Autodesk Inventor part; units mm, degrees
ref_plane "Work Plane1" through (0, 11.1125, 0) normal (0, 1, 0) x (-1, 0, 0)
ref_plane "YZ Plane" through (0, 0, 0) normal (1, 0, 0) x (0, 1, 0)
ref_plane "XY Plane" through (0, 0, 0) normal (0, 0, 1) x (1, 0, 0)
sketch "Sketch1" plane through (0, 0, 0) normal (0, 0, 1) x (1, 0, 0)
  circle A0 centre (0, 0) radius 11.1125
  circle A1 centre (0, 0) radius 5.5245
  circle A2 centre (0, 0) radius 1.8415
  dimension "d0" = 22.225
  dimension "d1" = 11.049
  dimension "d2" = 3.683
extrude "Extrusion1" add sketch "Sketch1" along normal blind 10.16 contours A0
extrude "Extrusion2" add sketch "Sketch1" along normal blind 5.08 contours A1
sketch "Sketch2" plane through (0, 0, 0) normal (1, 0, 0) x (0, 1, 0)
  line L0 (11.1125, 10.16) -> (-11.1125, 10.16)
  line L1 (2.8575, 10.16) -> (-2.8575, 10.16)
  line L2 (-2.8575, 10.16) -> (-2.8575, 6.096)
  line L3 (-2.8575, 6.096) -> (2.8575, 6.096)
  line L4 (2.8575, 6.096) -> (2.8575, 10.16)
  point P0 (0, 0)
  dimension "d7" = 5.715
  dimension "d8" = 2.8575
  dimension "d9" = 4.064
extrude "Extrusion3" cut sketch "Sketch2" along normal through all
ref_plane "Work Plane1" through (0, 11.1125, 0) normal (0, 1, 0) x (-1, 0, 0)
sketch "Sketch3" plane through (0, 11.1125, 0) normal (0, 1, 0) x (-1, 0, 0)
  line L0 (11.1125, 0) -> (11.1125, 10.16) construction
  circle A0 centre (0, 2.54) radius 1.7145
  point P0 (0, 0)
  dimension "d12" = 3.429
  dimension "d13" = 2.54
extrude "Extrusion4" cut sketch "Sketch3" against normal blind 2.032
pattern_circular "Circular Pattern1" count 4 over 360 about axis through (0, 0, 0) along (0, 0, 1) of "Extrusion4"
equation "\"d5\" = 0.5 * d3"
equation "\"d10\" = 0.5 * d3"
properties part number "EncoderDisc" material "ABS Plastic"
The model under review builds one solid part; all positions refer to its coordinate system, in mm. A direction names the side the tool comes from. Coordinates: 2 decimals unless noted, no trailing zeros. Loops run counter-clockwise (first coordinate to the right, second up) from the corner with the lowest first, then second, coordinate; pieces in that order, holes last. Notation, with made-up numbers: (6.25, 81.5) -> (11.25, 81.5) arc R28 ccw to (11.25, 106.5) -> close; hole circle Ø11 at (-8.75, 71.5). An arc over 180 degrees is marked (long way). Use a Markdown table: item, result. Add a question column.
1. To check wall thickness, follow line 1 (Z direction, x = 0, y = -10.25); line 2 (Z direction, x = 10.2, y = 0); line 3 (Z direction, x = 2.25, y = 4.25). State the ranges of each line that lie inside material, in increasing order.
2. Add section C-C on y = -5.25. Write out the cut boundary in (x, z), plus the area to 3 significant figures.
3. Add section A-A on x = 0. Write out the cut boundary in (y, z), plus the area to 3 significant figures.
4. Machinability: for faces 1 (the face through (8, -2.858, 8)), 2 (the face through (-10.111, 1.713, 2.615)), 3 (the face through (-1.713, -10.111, 2.615)), 4 (the face through (10.111, -1.713, 2.615)), which of the approach directions +Z, -Z, +X, -X, +Y, -Y give a long, thin tool a straight path to every point of the face, cutting with its end or side? Answer none if there is none.
5. Clearance check with flat-ended pins moving along their axes: pin 1 Ø12 at (x, y) = (-1, -2.5) entering from +Z; pin 2 Ø6 at (x, y) = (0, 0) entering from +Z; pin 3 Ø3.5 at (x, z) = (8, 8.5) entering from -Y; pin 4 Ø1 at (y, z) = (0.5, 3) entering from +X. State where each tip first meets the part, or that it passes through.
6. Add section D-D on z = 9.5. Write out the cut boundary in (x, y) (1 decimal).
7. Add section B-B on z = 1.5. Write out the cut boundary in (x, y) (1 decimal).
8. Draft analysis for pull direction X (two halves, no side actions). For faces 5 (the face through (10.265, 4.256, 5.009)), 6 (the face through (0, 9.08, 3)), 7 (the face through (-5.2, -2.3, 10.16)), state which applies: pulls with the +X half, pulls with the -X half, needs draft (parallel to the pull), parting line crosses it, or undercut.
Returned:
| question | item | result |
|---|---|---|
| 1 | line 1 | z = 0 to 0.83, 4.25 to 10.16 |
| 1 | line 2 | z = 0 to 0.83, 4.25 to 6.1 |
| 1 | line 3 | z = 0 to 5.08 |
| 2 | outline | (-9.79, 0) -> (9.79, 0) -> (9.79, 10.16) -> (1.72, 10.16) -> (1.72, 5.08) -> (-1.72, 5.08) -> (-1.72, 10.16) -> (-9.79, 10.16) -> close |
| 2 | area | 182 mm² |
| 3 | outline | (-11.11, 0) -> (-1.84, 0) -> (-1.84, 5.08) -> (-5.52, 5.08) -> (-5.52, 10.16) -> (-11.11, 10.16) -> (-11.11, 4.25) -> (-9.08, 4.25) -> (-9.08, 0.83) -> (-11.11, 0.83) -> close; (1.84, 0) -> (11.11, 0) -> (11.11, 0.83) -> (9.08, 0.83) -> (9.08, 4.25) -> (11.11, 4.25) -> (11.11, 10.16) -> (5.52, 10.16) -> (5.52, 5.08) -> (1.84, 5.08) -> close |
| 3 | area | 137 mm² |
| 4 | face 1 | +Z, +X |
| 4 | face 2 | -X |
| 4 | face 3 | -Y |
| 4 | face 4 | +X |
| 5 | pin 1 | stops at z = 10.16 |
| 5 | pin 2 | stops at z = 5.08 |
| 5 | pin 3 | stops at y = -9.19 |
| 5 | pin 4 | stops at x = 9.08 |
| 6 | outline | (4.7, -2.9) arc R5.5 cw (long way) to (4.7, 2.9) -> (10.7, 2.9) arc R11.1 ccw (long way) to (10.7, -2.9) -> close |
| 7 | outline | (-11, -1.4) arc R11.1 ccw to (-1.4, -11) -> (-1.4, -9.1) -> (1.4, -9.1) -> (1.4, -11) arc R11.1 ccw to (11, -1.4) -> (9.1, -1.4) -> (9.1, 1.4) -> (11, 1.4) arc R11.1 ccw to (1.4, 11) -> (1.4, 9.1) -> (-1.4, 9.1) -> (-1.4, 11) arc R11.1 ccw to (-11, 1.4) -> (-9.1, 1.4) -> (-9.1, -1.4) -> close; hole circle Ø3.7 at (0, 0) |
| 8 | face 5 | parting line crosses it |
| 8 | face 6 | undercut |
| 8 | face 7 | needs draft |
